Input: part model. Units: mm. Frame: model coordinates. A direction names the side the tool comes from. Coordinates: 2 decimals unless noted, no trailing zeros. Order: outer loops, then holes, each group sorted by start corner. A loop starts at its lowest first (then second) coordinate and runs counter-clockwise, first axis right, second up. Notation, with made-up numbers: (40.5, -20.75) -> (75.5, -20.75) arc R11 ccw to (75.5, -7.75) -> close; hole circle Ø10 at (39, 13.5). An arc over 180 degrees is marked (long way). One line per item, written item: value. Start each with the question number.
from build123d import *

# Parameters (mm, degrees)
ESBO_O1_R                = 1
ESBO_O1_R_2              = 3.5
RESSALTO_EXTRUS_O1_DEPTH = 3
FILETE1_R                = 20


with BuildPart() as part:
    # Esboço1 → Ressalto-extrusão1 (new body)
    with BuildSketch(Plane.XY):
        with BuildLine():
            Line((5.590169944, -5), (54.409830056, -5))
            ThreePointArc((54.409830056, -5), (67.5, 0), (54.409830056, 5))
            Line((54.409830056, 5), (5.590169944, 5))
            ThreePointArc((5.590169944, 5), (-7.5, 0), (5.590169944, -5))
        make_face()
        with Locations((44, 0)):
            Circle(ESBO_O1_R, mode=Mode.SUBTRACT)
        with Locations((16, 0)):
            Circle(ESBO_O1_R, mode=Mode.SUBTRACT)
        Circle(ESBO_O1_R_2, mode=Mode.SUBTRACT)
        with Locations((60, 0)):
            Circle(ESBO_O1_R_2, mode=Mode.SUBTRACT)
        with BuildLine():
            Line((30.901387819, 1.5), (36.5, 1.5))
            Line((36.5, 1.5), (36.5, -1.5))
            Line((36.5, -1.5), (30.901387819, -1.5))
            ThreePointArc((30.901387819, -1.5), (30, -1.75), (29.098612181, -1.5))
            Line((29.098612181, -1.5), (23.5, -1.5))
            Line((23.5, -1.5), (23.5, 1.5))
            Line((23.5, 1.5), (29.098612181, 1.5))
            ThreePointArc((29.098612181, 1.5), (30, 1.75), (30.901387819, 1.5))
        make_face(mode=Mode.SUBTRACT)
    extrude(amount=RESSALTO_EXTRUS_O1_DEPTH)

    # Filete1
    filete1_edges = [part.edges().sort_by_distance(p)[0] for p in [
        (54.409830056, -5, 1.5),
        (5.590169944, -5, 1.5),
        (5.590169944, 5, 1.5),
        (54.409830056, 5, 1.5),
    ]]
    fillet(filete1_edges, radius=FILETE1_R)


solid = part.part
1) Section query A-A, the plane x = 28. Return the cut outline in (y, z), plus the area to 3 significant figures.
2) Pin query (flat end, axial travel): pin 1 Ø0.9 at (x, z) = (28, 1.5) entering from -Y; pin 2 Ø0.9 at (x, z) = (33.5, 1) entering from +Y. Return the tip coordinate at first contact, or that it passes through.
3) Access query for faces 1 (the flat face through (34, -1.5, 1)), 2 (the cylindrical face through (52.866, 5.473, 1.521)), 3 (the flat face through (29, 2, 3)). Directions: +Z, -Z, +X, -X, +Y, -Y. A direction counts if a zero-diameter tool reaches every point of the face in a straight line with its end or side. Return the directions, or none.
4) Mould query, pull axis Y, two halves, no side actions, for faces 4 (the flat face through (30, -5, 1)), 5 (the flat face through (30, 5, 1)), 6 (the cylindrical face through (67.497, -0.21, 1.479)), 7 (the flat face through (26, -1.5, 1)). Classes: +Y half, -Y half, draft (parallel to the pull), parting line (faces both ways), or undercut.
5) Section query D-D, the plane x = 44. Return the cut outline in (y, z).
6) Section query C-C, the plane z = 1.7. Return the cut outline in (x, y), plus the area to 3 significant figures.
7) Ray query, line 1 along Y through (x, z) = (60, 0.8); line 2 along Y through (x, z) = (44, 1.05); line 3 along X through (y, z) = (-2.5, 1.4). Return the intervals inside material, ascending. Write a range as from..to.
8) Section query B-B, the plane y = 0. Return the cut outline in (x, z).
Entries:
1. outline: (-5, 0) -> (-1.5, 0) -> (-1.5, 3) -> (-5, 3) -> close; (1.5, 0) -> (5, 0) -> (5, 3) -> (1.5, 3) -> close
1. area: 21.0 mm2
2. pin 1: stops at y = -5
2. pin 2: stops at y = 5
3. face 1: +Z, -Z
3. face 2: +Z, -Z, +Y
3. face 3: +Z, +X, -X, +Y, -Y
4. face 4: -Y half
4. face 5: +Y half
4. face 6: parting line
4. face 7: undercut
5. outline: (-5, 0) -> (-1, 0) -> (-1, 3) -> (-5, 3) -> close; (1, 0) -> (5, 0) -> (5, 3) -> (1, 3) -> close
6. outline: (3.12, -6.82) arc R20 cw to (11.46, -5) -> (48.54, -5) arc R20 cw to (56.88, -6.82) arc R7.5 ccw (long way) to (56.88, 6.82) arc R20 cw to (48.54, 5) -> (11.46, 5) arc R20 cw to (3.12, 6.82) arc R7.5 ccw (long way) to start; hole circle Ø7 at (0, 0); hole circle Ø2 at (16, 0); hole (23.5, -1.5) -> (29.1, -1.5) arc R1.75 ccw to (30.9, -1.5) -> (36.5, -1.5) -> (36.5, 1.5) -> (30.9, 1.5) arc R1.75 ccw to (29.1, 1.5) -> (23.5, 1.5) -> close; hole circle Ø2 at (44, 0); hole circle Ø7 at (60, 0)
6. area: 702 mm2
7. line 1: y = -7.5..-3.5, 3.5..7.5
7. line 2: y = -5..-1, 1..5
7. line 3: x = -7.07..-2.45, 2.45..57.55, 62.45..67.07
8. outline: (-7.5, 0) -> (-3.5, 0) -> (-3.5, 3) -> (-7.5, 3) -> close; (3.5, 0) -> (15, 0) -> (15, 3) -> (3.5, 3) -> close; (17, 0) -> (23.5, 0) -> (23.5, 3) -> (17, 3) -> close; (36.5, 0) -> (43, 0) -> (43, 3) -> (36.5, 3) -> close; (45, 0) -> (56.5, 0) -> (56.5, 3) -> (45, 3) -> close; (63.5, 0) -> (67.5, 0) -> (67.5, 3) -> (63.5, 3) -> close
